Check sheet for the modelled part. Datum: model origin and axes. Units: mm. Round coordinates to 2 decimals unless told otherwise and drop trailing zeros. Write each loop counter-clockwise with the first axis right and the second up, starting at its lowest first coordinate (ties: lowest second). Pieces come first, ordered by that corner, then holes. Notation, with made-up numbers: M 50.5,62.25 L 87.5,62.25 A30 cw 87.5,99.25 Z; hole C 69,72 d10. An arc over 180 degrees is marked long. One line per item, written item: value.
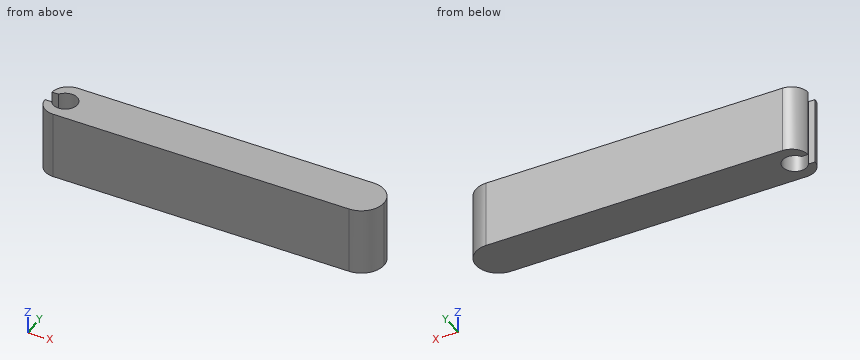
from build123d import *

# Parameters (mm, degrees)
ESQUISSE1_W                  = 60
ESQUISSE1_H                  = 8
BOSS_EXTRU_1_DEPTH           = 12
ENL_V_MAT_EXTRU_1_DEPTH      = 62.708994482
ENL_V_MAT_EXTRU_1_DEPTH_BACK = 62.708994482
ESQUISSE2_R                  = 2.15
ENL_V_MAT_EXTRU_2_DEPTH      = 62.708994482
ENL_V_MAT_EXTRU_2_DEPTH_BACK = 62.708994482
ESQUISSE3_W                  = 2
ESQUISSE3_H                  = 2.3
CONG_1_R                     = 4
CONG_2_R                     = 3


# Some blends are built 0.0001 mm under size
with BuildPart() as part:
    # Esquisse1 → Boss.-Extru.1 (new body)
    with BuildSketch(Plane.XY):
        with Locations((30, 4)):
            Rectangle(ESQUISSE1_W, ESQUISSE1_H)
    extrude(amount=BOSS_EXTRU_1_DEPTH)

    # Esquisse2 → Enlèv. mat.-Extru.1 (cut, two sides: drawn at the far end of the back side and taken through both)
    with BuildSketch(Plane.XY.offset(12).offset(-ENL_V_MAT_EXTRU_1_DEPTH_BACK)):
        with Locations((3, 4)):
            Circle(ESQUISSE2_R)
    extrude(amount=ENL_V_MAT_EXTRU_1_DEPTH + ENL_V_MAT_EXTRU_1_DEPTH_BACK, mode=Mode.SUBTRACT)

    # Esquisse3 → Enlèv. mat.-Extru.2 (cut, two sides: drawn at the far end of the back side and taken through both)
    with BuildSketch(Plane.XY.offset(12).offset(-ENL_V_MAT_EXTRU_2_DEPTH_BACK)):
        with Locations((1, 4)):
            Rectangle(ESQUISSE3_W, ESQUISSE3_H)
    extrude(amount=ENL_V_MAT_EXTRU_2_DEPTH + ENL_V_MAT_EXTRU_2_DEPTH_BACK, mode=Mode.SUBTRACT)

    # Congé1
    cong_1_edges = [part.edges().sort_by_distance(p)[0] for p in [
        (60, 0, 6),
        (60, 8, 6),
    ]]
    fillet(cong_1_edges, radius=CONG_1_R - 0.0001)  # a hair under: the kernel refuses the full size

    # Congé2
    # the kernel refuses this fillet: 3 mm, written as the material it takes off along each edge
    with BuildSketch(Plane(origin=(0, 0, -7.490619133), x_dir=(1, 0, 0), z_dir=(0, 0, 1))) as cong_2_piece_1:
        with BuildLine():
            CenterArc((2.996247653, 3), CONG_2_R, 182.865983983, 87.134016017)
            Line((0, 2.85), (-0.059924953, 2.847))
            ThreePointArc((-0.059924953, 2.847), (-0.06, 1.425), (-0.06, 0))
            Line((-0.06, 0), (0, -0.06))
            Line((0, -0.06), (2.996247653, -0.06))
            Line((2.996247653, -0.06), (2.996247653, 0))
        make_face()
    extrude(amount=26.981238267, mode=Mode.SUBTRACT)
    with BuildSketch(Plane(origin=(0, 8, -7.490619133), x_dir=(1, 0, 0), z_dir=(0, 0, 1))) as cong_2_piece_2:
        with BuildLine():
            CenterArc((2.996247653, -3), CONG_2_R, 90, 87.134016017)
            Line((0, -2.85), (-0.059924953, -2.847))
            ThreePointArc((-0.059924953, -2.847), (-0.06, -1.425), (-0.06, 0))
            Line((-0.06, 0), (0, 0.06))
            Line((0, 0.06), (2.996247653, 0.06))
            Line((2.996247653, 0.06), (2.996247653, 0))
        make_face()
    extrude(amount=26.981238267, mode=Mode.SUBTRACT)


solid = part.part
Q1. Sectioned sample at C-C on y = 3.5. Enter the section's corners in (x, z), and give its area (3 significant figures).
Completed:
outline: M 5.09,0 L 59.97,0 L 59.97,12 L 5.09,12 Z
area: 659 mm^2
Q2. Scan lines: line 1 (Y direction, x = 3, z = 4.25); line 2 (X direction, y = 5.75, z = 11); line 3 (X direction, y = 4, z = 5.75). Record each from-to range of solid material in increasing order. Write a range as [from, to].
Completed:
line 1: [0, 1.85], [6.15, 8]
line 2: [0.09, 1.75], [4.25, 59.6]
line 3: [5.15, 60]
Q3. Sectioned sample at B-B on y = 6.75. Enter the section's corners in (x, z), and give its area (3 significant figures).
Completed:
outline: M 0.56,0 L 58.9,0 L 58.9,12 L 0.56,12 Z
area: 700 mm^2
Q4. Depth check by flat-ended pin: P1, Ø0.9, axis at x = 0.5, z = 9, coming from the +Y side; P2, Ø0.6, axis at x = 0.5, z = 4.5, coming from the -Y side. Enter the tip coordinate at first touch or a pass-through.
Completed:
P1: y = 7.19
P2: y = 0.96
